```python
from build123d import *

# Parameters (mm, degrees)
SKETCH1_W           = 54
SKETCH1_H           = 94
BOSS_EXTRUDE1_DEPTH = 4
CUT_EXTRUDE1_REACH  = 6
SKETCH2_W           = 2
SKETCH2_H           = 10
SKETCH3_R           = 1.25
CUT_EXTRUDE2_DEPTH  = 5
CHAMFER1_SIZE       = 1
SKETCH4_R           = 2
CUT_EXTRUDE3_DEPTH  = 2


with BuildPart() as part:
    # Sketch1 → Boss-Extrude1 (new body)
    with BuildSketch(Plane.XY):
        with Locations((27, 47)):
            Rectangle(SKETCH1_W, SKETCH1_H)
    extrude(amount=BOSS_EXTRUDE1_DEPTH)

    # Sketch2 → Cut-Extrude1 (cut, up to next)
    with BuildSketch(Plane.XY.offset(4), mode=Mode.PRIVATE) as cut_extrude1_sk1:
        with Locations((1, 47)):
            Rectangle(SKETCH2_W, SKETCH2_H)
    cut_extrude1_tool1 = extrude(cut_extrude1_sk1.sketch, amount=-CUT_EXTRUDE1_REACH, mode=Mode.PRIVATE) & part.part
    add(cut_extrude1_tool1.solids().sort_by_distance((1, 47, 4))[0], mode=Mode.SUBTRACT)

    # Sketch3 → Cut-Extrude2 (cut, through all)
    with BuildSketch(Plane.XY.offset(4)):
        with Locations((27, 89)):
            Circle(SKETCH3_R)
        with Locations((27, 5)):
            Circle(SKETCH3_R)
    extrude(amount=-CUT_EXTRUDE2_DEPTH, mode=Mode.SUBTRACT)

    # Chamfer1
    chamfer1_edges = [part.edges().sort_by_distance(p)[0] for p in [
        (2, 47, 0),
    ]]
    chamfer(chamfer1_edges, length=CHAMFER1_SIZE)

    # Sketch4 → Cut-Extrude3 (cut)
    with BuildSketch(Plane.XY.offset(4)):
        with Locations((27, 89)):
            Circle(SKETCH4_R)
        with Locations((27, 5)):
            Circle(SKETCH4_R)
    extrude(amount=-CUT_EXTRUDE3_DEPTH, mode=Mode.SUBTRACT)


solid = part.part
```
Design review of the part built by this model. Coordinates are the model's own, in mm. A direction names the side the tool comes from. Round coordinates to 2 decimals unless told otherwise and drop trailing zeros. Order: outer loops, then holes, each group sorted by start corner. A loop starts at its lowest first (then second) coordinate and runs counter-clockwise, first axis right, second up. Notation, with made-up numbers: M -33.75,63 L 5.25,63 A15 ccw 5.25,89 Z; hole C 69.25,1 d3. An arc over 180 degrees is marked long. Put each result on its own line as item: value.
Q1. Machinability: for faces 5 (the face through (28, 90, 2)), 6 (the face through (27, 48, 4)), which of the approach directions +Z, -Z, +X, -X, +Y, -Y give a long, thin tool a straight path to every point of the face, cutting with its end or side? Answer none if there is none.
Reported:
face 5: +Z
face 6: +Z, +X, -X, +Y, -Y
Q2. Consider section B-B (y = 89). State the section outline as (x, z) points.
Reported:
outline: M 0,0 L 25.75,0 L 25.75,2 L 25,2 L 25,4 L 0,4 Z; M 28.25,0 L 54,0 L 54,4 L 29,4 L 29,2 L 28.25,2 Z
Q3. Insertion check: pin 1 Ø3 at (x, y) = (27, 89) entering from +Z; pin 2 Ø1.5 at (y, z) = (44.5, 2) entering from -X. Each pin has a flat end and moves straight along its axis. Give the tip position at first contact, or say it passes through.
Reported:
pin 1: z = 2
pin 2: x = 2
Q4. Consider section A-A (x = 27). State the section outline as (y, z) points, and give its area (3 significant figures).
Reported:
outline: M 0,0 L 3.75,0 L 3.75,2 L 3,2 L 3,4 L 0,4 Z; M 6.25,0 L 87.75,0 L 87.75,2 L 87,2 L 87,4 L 7,4 L 7,2 L 6.25,2 Z; M 90.25,0 L 94,0 L 94,4 L 91,4 L 91,2 L 90.25,2 Z
area: 350 mm²
Q5. Draft analysis for pull direction X (two halves, no side actions). For faces 1 (the face through (54, 46, 2)), 2 (the face through (28.908, 5.601, 3.014)), 3 (the face through (2, 47, 3)), 4 (the face through (1, 42, 2)), state which applies: released by +X, released by -X, zero draft, split by the parting line, or undercut.
Reported:
face 1: released by +X
face 2: undercut
face 3: released by -X
face 4: zero draft
Q6. To check wall thickness, follow line 1 (Y direction, x = 27, z = 2.85); line 2 (Y direction, x = 27, z = 1); line 3 (X direction, y = 89, z = 1). State the ranges of each line that lie inside material, in increasing order.
Reported:
line 1: 0 to 3, 7 to 87, 91 to 94
line 2: 0 to 3.75, 6.25 to 87.75, 90.25 to 94
line 3: 0 to 25.75, 28.25 to 54
